The listing builds one solid part. Answer for the finished solid, in the listing's coordinates (mm). Face numbers are marked on the shaded views. A direction names the side the tool comes from. Give positions to 0.01 mm unless a question says otherwise; leave off trailing zeros. Order: outer loops, then holes, each group sorted by start corner. A loop starts at its lowest first (then second) coordinate and runs counter-clockwise, first axis right, second up. Notation, with made-up numbers: M 50.5,22.25 L 83.5,22.25 A14 cw 83.5,49.25 Z; hole C 68.25,22 d9. An arc over 180 degrees is marked long. Answer as a JSON object with one key per item and string values. Group by question number.
```python
from build123d import *

# Parameters (mm, degrees)
SKETCH1_R           = 30
SKETCH1_R_2         = 15
BOSS_EXTRUDE1_DEPTH = 10
SKETCH2_R           = 30
BOSS_EXTRUDE2_DEPTH = 10
FILLET1_R           = 10


with BuildPart() as part:
    # Sketch1 → Boss-Extrude1 (new body)
    with BuildSketch(Plane(origin=(0, 0, 0), x_dir=(1, 0, 0), z_dir=(0, 1, 0))):
        Circle(SKETCH1_R)
        with BuildLine():
            ThreePointArc((2.5, 24.874685928), (0, -25), (-2.5, 24.874685928))
            Line((-2.5, 24.874685928), (-2.5, 19.843134833))
            ThreePointArc((-2.5, 19.843134833), (0, -20), (2.5, 19.843134833))
            Line((2.5, 19.843134833), (2.5, 24.874685928))
        make_face(mode=Mode.SUBTRACT)
        Circle(SKETCH1_R_2, mode=Mode.SUBTRACT)
    extrude(amount=BOSS_EXTRUDE1_DEPTH)

    # Sketch2 → Boss-Extrude2 (add)
    with BuildSketch(Plane(origin=(0, 10, 0), x_dir=(1, 0, 0), z_dir=(0, 1, 0))):
        Circle(SKETCH2_R)
    extrude(amount=BOSS_EXTRUDE2_DEPTH)

    # Fillet1
    fillet1_edges = [part.edges().sort_by_distance(p)[0] for p in [
        (-30, 20, 0),
    ]]
    fillet(fillet1_edges, radius=FILLET1_R)


solid = part.part
```
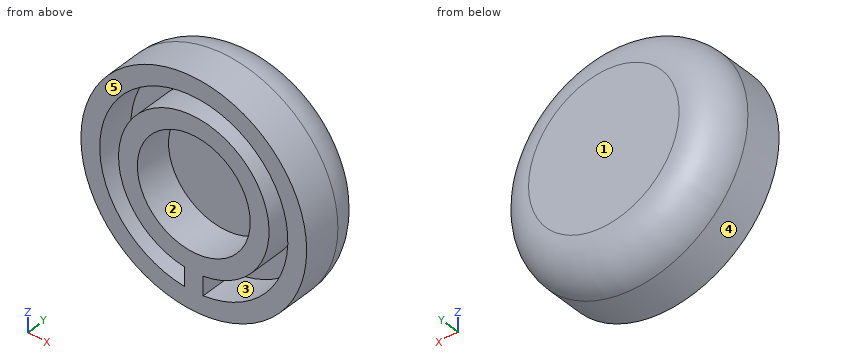
Item 1: A tool of negligible diameter and unlimited length cuts with its end or side. For the marked faces 1 and 2, from which of +Z, -Z, +X, -X, +Y, -Y can it reach the whole face along a straight path? Write none if from no direction.
Item 2: Determine the mould class of the marked faces 3, 4 and 5 for opening direction Z: released by +Z, released by -Z, zero draft, split by the parting line, or undercut.
Item 3: Flat-ended cylindrical pins translate along their axes: P1, Ø12, axis at x = -16.5, y = 16, coming from the -Z side; P2, Ø1.5, axis at y = 11, z = 11, coming from the +X side; P3, Ø4, axis at y = 15.5, z = 7, coming from the +X side; P4, Ø4, axis at x = -12, z = -11.5, coming from the -Y side. Find the tip coordinate at first contact, or state that the pin passes through.
Item 4: Section C-C (y = 15.75) is taken. Determine the outline of the cut face in (x, z), and give its area (3 significant figures).
Item 5: Section A-A (x = 0) is taken. Determine the outline of the cut face in (y, z), and give its area (3 significant figures).
Item 6: Section B-B (z = 0) is taken. Determine the outline of the cut face in (x, y), and give its area (3 significant figures).
Item 7: Consider probe 1 along X at (y, z) = (6.75, 0); probe 2 along X at (y, z) = (5.25, -2); probe 3 along X at (y, z) = (3.5, -20.5). Determine where each line is inside the solid, lowest interval first. Write a range as from..to.
Values found:
{
 "1": {"face 1": "+Z, -Z, +X, -X, +Y", "face 2": "-Y"},
 "2": {"face 3": "undercut", "face 4": "split by the parting line", "face 5": "zero draft"},
 "3": {"P1": "stops at z = -27.31", "P2": "stops at x = 28.15", "P3": "stops at x = 28.64", "P4": "stops at y = 0"},
 "4": {"outline": "C 0,0 d56.36", "area": "2,500 mm^2"},
 "5": {"outline": "M 0,-30 L 10,-30 A10 ccw 20,-20 L 20,20 A10 ccw 10,30 L 0,30 L 0,25 L 10,25 L 10,20 L 0,20 L 0,15 L 10,15 L 10,-15 L 0,-15 Z", "area": "807 mm^2"},
 "6": {"outline": "M -30,0 L -25,0 L -25,10 L -20,10 L -20,0 L -15,0 L -15,10 L 15,10 L 15,0 L 20,0 L 20,10 L 25,10 L 25,0 L 30,0 L 30,10 A10 ccw 20,20 L -20,20 A10 ccw -30,10 Z", "area": "757 mm^2"},
 "7": {"probe 1": "x = -30..-25, -20..-15, 15..20, 25..30", "probe 2": "x = -29.93..-24.92, -19.9..-14.87, 14.87..19.9, 24.92..29.93", "probe 3": "x = -21.9..-14.31, -2.5..2.5, 14.31..21.9"}
}
